Can you work these out from the drawing? Everything is in mm from the part's minimum corner. A direction names the side the tool comes from. Give positions to 0.01 mm unless a question says otherwise; leave off trailing zeros. Loops run counter-clockwise (first coordinate to the right, second up) from the corner with the lowest first, then second, coordinate; pieces in that order, holes last. Notation, with made-up numbers: (29.25, 2.25) -> (88.25, 2.25) arc R26 cw to (88.25, 34.25) -> close; hole circle Ø3 at (-35.5, -28). An arc over 180 degrees is marked (long way). Return JSON: item names as keys, results as strings. Group by question number.
Q1. Suppose I cut it at D-D, the plane y = 19. Please give me the cut outline in (x, z), and give its area (3 significant figures).
Q2. Suppose I cut it at A-A, the plane y = 65. Please give me the cut outline in (x, z), and give its area (3 significant figures).
Q3. Which directions (+Z, -Z, +X, -X, +Y, -Y) give clear straight access to the entire face, cutting with the end or side of a thin tool? Please do the marked faces 5, 6 and 7.
Q4. Thinking about a two-plate mould opening in Z: for the marked faces 1, 2, 3 and 4, which applies, pulls with the +Z half, pulls with the -Z half, needs draft (parallel to the pull), parting line crosses it, or undercut?
Q5. Will these pins go through, and if not, where does the flat tip stop? pin 1 (22 mm diameter, centred on y = 65, z = 50, fed in from -X); pin 2 (6 mm diameter, centred on x = 17, z = 81.5, fed in from +Y); pin 3 (21 mm diameter, centred on y = 36, z = 37, fed in from +X); pin 4 (4 mm diameter, centred on y = 63, z = 45.5, fed in from -X).
Q6. I need wall thicknesses on line 1 along Y through (x, z) = (46.75, 50); line 2 along Y through (x, z) = (70, 24.5); line 3 along X through (y, z) = (31.5, 51). Which ranges of each line are inside material? Lowest first, please. Write a range as [from, to].
Q7. Suppose I cut it at C-C, the plane z = 55. Please give me the cut outline in (x, y).
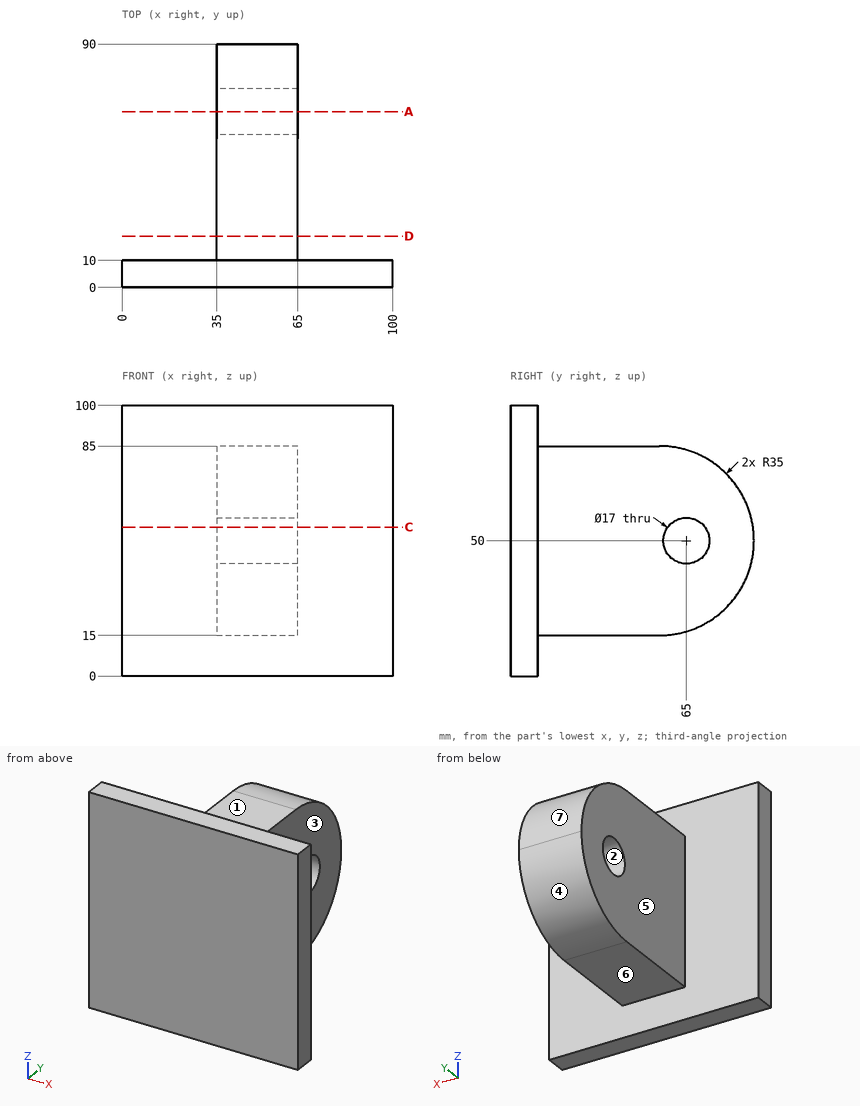
Ans:
{
 "1": {"outline": "(35, 15) -> (65, 15) -> (65, 85) -> (35, 85) -> close", "area": "2,100 mm^2"},
 "2": {"outline": "(35, 16.46) -> (65, 16.46) -> (65, 41.5) -> (35, 41.5) -> close; (35, 58.5) -> (65, 58.5) -> (65, 83.54) -> (35, 83.54) -> close", "area": "1,500 mm^2"},
 "3": {"face 5": "+Z, -Z, -X, +Y", "face 6": "-Z, +X, -X, +Y", "face 7": "+Z, +X, -X, +Y"},
 "4": {"face 1": "pulls with the +Z half", "face 2": "undercut", "face 3": "needs draft", "face 4": "pulls with the -Z half"},
 "5": {"pin 1": "stops at x = 35", "pin 2": "stops at y = 10", "pin 3": "stops at x = 65", "pin 4": "passes through"},
 "6": {"line 1": "y = [0, 56.5], [73.5, 90]", "line 2": "y = [0, 10]", "line 3": "x = [35, 65]"},
 "7": {"outline": "(0, 0) -> (100, 0) -> (100, 10) -> (65, 10) -> (65, 58.13) -> (35, 58.13) -> (35, 10) -> (0, 10) -> close; (35, 71.87) -> (65, 71.87) -> (65, 89.64) -> (35, 89.64) -> close"}
}
